```python
from build123d import *

# Parameters (mm, degrees)
F1_DEPTH = 31.75


with BuildPart() as f1:
    # F0 (on Front) → F1 (new body)
    with BuildSketch(Plane.XZ):
        with BuildLine():
            Line((-24.867260192, 14.0561722352), (-20.5749857529, 14.0561722352))
            ThreePointArc((-20.5749857529, 14.0561722352), (-21.7302586773, 16.117381452), (-22.3627959644, 18.394031523))
            Line((-22.3627959644, 18.394031523), (-24.867260192, 14.0561722352))
        make_face()
        with BuildLine():
            ThreePointArc((-17.3257802935, 14.0561722352), (-19.3712146858, 16.6546470319), (-20.1002728939, 19.8802240735))
            Line((-20.1002728939, 19.8802240735), (-20.1002728939, 22.3128364345))
            Line((-20.1002728939, 22.3128364345), (-22.3627959644, 18.394031523))
            ThreePointArc((-22.3627959644, 18.394031523), (-21.7302586773, 16.117381452), (-20.5749857529, 14.0561722352))
            Line((-20.5749857529, 14.0561722352), (-17.3257802935, 14.0561722352))
        make_face()
        with BuildLine():
            Line((-22.3627959644, 18.394031523), (-20.1002728939, 22.3128364345))
            Line((-20.1002728939, 22.3128364345), (-20.1002728939, 26.3040566523))
            ThreePointArc((-20.1002728939, 26.3040566523), (-21.8625114192, 23.3046309565), (-22.4752728939, 19.8802240735))
            ThreePointArc((-22.4752728939, 19.8802240735), (-22.4471135121, 19.1350027378), (-22.3627959644, 18.394031523))
        make_face()
        with BuildLine():
            ThreePointArc((-22.4752728939, 19.8802240735), (-21.8625114192, 23.3046309565), (-20.1002728939, 26.3040566523))
            Line((-20.1002728939, 26.3040566523), (-20.1002728939, 30.2920383944))
            Line((-20.1002728939, 30.2920383944), (-22.4752728939, 30.2920383944))
            Line((-22.4752728939, 30.2920383944), (-22.4752728939, 19.8802240735))
        make_face()
        with BuildLine():
            ThreePointArc((-20.1002728939, 19.8802240735), (-12.6002728939, 27.3802240735), (-5.1002728939, 19.8802240735))
            Line((-5.1002728939, 19.8802240735), (-5.1002728939, 22.1484367352))
            Line((-5.1002728939, 22.1484367352), (-5.1002728939, 26.3040566523))
            ThreePointArc((-5.1002728939, 26.3040566523), (-12.6002728939, 29.7552240735), (-20.1002728939, 26.3040566523))
            Line((-20.1002728939, 26.3040566523), (-20.1002728939, 22.3128364345))
            Line((-20.1002728939, 22.3128364345), (-20.1002728939, 19.8802240735))
        make_face()
        with BuildLine():
            Line((-5.1002728939, 22.1484367352), (-5.1002728939, 19.8802240735))
            ThreePointArc((-5.1002728939, 19.8802240735), (-5.8293311021, 16.6546470319), (-7.8747654943, 14.0561722352))
            Line((-7.8747654943, 14.0561722352), (-4.6255600349, 14.0561722352))
            ThreePointArc((-4.6255600349, 14.0561722352), (-3.4953535559, 16.057127312), (-2.8582453868, 18.265131181))
            Line((-2.8582453868, 18.265131181), (-5.1002728939, 22.1484367352))
        make_face()
        with BuildLine():
            Line((-5.1002728939, 26.3040566523), (-5.1002728939, 22.1484367352))
            Line((-5.1002728939, 22.1484367352), (-2.8582453868, 18.265131181))
            ThreePointArc((-2.8582453868, 18.265131181), (-2.758572161, 19.0699453043), (-2.7252728939, 19.8802240735))
            ThreePointArc((-2.7252728939, 19.8802240735), (-3.3380343686, 23.3046309565), (-5.1002728939, 26.3040566523))
        make_face()
        with BuildLine():
            ThreePointArc((-2.8582453868, 18.265131181), (-3.4953535559, 16.057127312), (-4.6255600349, 14.0561722352))
            Line((-4.6255600349, 14.0561722352), (-0.4282018064, 14.0561722352))
            Line((-0.4282018064, 14.0561722352), (-2.8582453868, 18.265131181))
        make_face()
        with BuildLine():
            Line((-5.1002728939, 30.2920383944), (-5.1002728939, 26.3040566523))
            ThreePointArc((-5.1002728939, 26.3040566523), (-3.3380343686, 23.3046309565), (-2.7252728939, 19.8802240735))
            Line((-2.7252728939, 19.8802240735), (-2.7252728939, 30.2920383944))
            Line((-2.7252728939, 30.2920383944), (-5.1002728939, 30.2920383944))
        make_face()
    extrude(amount=F1_DEPTH)


solid = f1.part
```
Here's how the part is built. I have some questions about the finished solid (model axes, mm). A direction names the side the tool comes from. Round coordinates to 2 decimals unless told otherwise and drop trailing zeros. Write each loop counter-clockwise with the first axis right and the second up, starting at its lowest first coordinate (ties: lowest second). Pieces come first, ordered by that corner, then holes.
Q1. If we section it at C-C on x = -6.25: Write out the boundary of the cut face in (y, z), plus the area to 3 significant figures.
Q2. Will these pins go through, and if not, where does the flat tip stop? P1, Ø4.5, axis at y = -19.5, z = 28, coming from the +X side; P2, Ø5, axis at x = -14.5, y = -6.5, coming from the -Z side; P3, Ø3, axis at y = -28, z = 17.5, coming from the -X side (3 decimals).
Q3. If we section it at D-D on z = 28.75: Write out the boundary of the cut face in (x, y), plus the area to 3 significant figures.
Q4. If we mould it in two halves opening along X, with no side actions, what happens to faces 1 (the flat face through (-12, 0, 28)), 2 (the flat face through (-22.475, -16, 25)), 3 (the flat face through (-5.1, -16, 28))? For each: +X half, -X half, draft (parallel to the pull), parting line (faces both ways), or undercut.
Q5. If we section it at A-A on z = 20.5: Write out the boundary of the cut face in (x, y), plus the area to 3 significant figures.
Q6. Which directions (+Z, -Z, +X, -X, +Y, -Y) give clear straight access to the entire face, cutting with the end or side of a thin tool? Please do faces 4 (the cylindrical face through (-2.76, -15.65, 19.06)), 5 (the cylindrical face through (-22.45, -15.65, 19.15)), 6 (the flat face through (-20.1, -16, 28)).
Q7. If we section it at B-B on y = -5: Write out the boundary of the cut face in (x, z) (3 decimals).
Q8. Please list where these lines run through material, in increasing order: probe 1 along X at (y, z) = (-22.5, 21.5); probe 2 along X at (y, z) = (-6.5, 28.5); probe 3 along X at (y, z) = (-5, 20.25).
Answer below:
1. outline: (-31.75, 14.06) - (0, 14.06) - (0, 15.89) - (-31.75, 15.89) - close; (-31.75, 23.87) - (0, 23.87) - (0, 27.44) - (-31.75, 27.44) - close
1. area: 172 mm2
2. P1: stops at x = -2.73
2. P2: stops at z = 25.95
2. P3: stops at x = -23.745
3. outline: (-22.48, -31.75) - (-20.1, -31.75) - (-20.1, 0) - (-22.48, 0) - close; (-16.94, -31.75) - (-8.26, -31.75) - (-8.26, 0) - (-16.94, 0) - close; (-5.1, -31.75) - (-2.73, -31.75) - (-2.73, 0) - (-5.1, 0) - close
3. area: 426 mm2
4. face 1: draft
4. face 2: -X half
4. face 3: undercut
5. outline: (-22.48, -31.75) - (-20.07, -31.75) - (-20.07, 0) - (-22.48, 0) - close; (-5.13, -31.75) - (-2.73, -31.75) - (-2.73, 0) - (-5.13, 0) - close
5. area: 152 mm2
6. face 4: +X, +Y, -Y
6. face 5: -X, +Y, -Y
6. face 6: +Z, +Y, -Y
7. outline: (-24.867, 14.056) - (-17.326, 14.056) arc R7.5 cw (long way) to (-7.875, 14.056) - (-0.428, 14.056) - (-2.858, 18.265) arc R9.875 ccw to (-2.725, 19.88) - (-2.725, 30.292) - (-5.1, 30.292) - (-5.1, 26.304) arc R9.875 ccw to (-20.1, 26.304) - (-20.1, 30.292) - (-22.475, 30.292) - (-22.475, 19.88) arc R9.875 ccw to (-22.363, 18.394) - close
8. probe 1: x = -22.48 to -19.92, -5.28 to -2.73
8. probe 2: x = -22.48 to -20.1, -17.42 to -7.78, -5.1 to -2.73
8. probe 3: x = -22.48 to -20.09, -5.11 to -2.73
